The figure shows three views and two pictorial views of one solid part (mm, origin at its lowest corner). Answer the questions. Give positions to 0.01 mm unless a question says otherwise; leave off trailing zeros. Loops run counter-clockwise (first coordinate to the right, second up) from the corner with the lowest first, then second, coordinate; pieces in that order, holes last. Notation, with made-up numbers: (15.25, 34) -> (24.25, 34) arc R30 ccw to (24.25, 56) -> close; hole circle Ø5 at (57, 83.25). An arc over 180 degrees is marked (long way). Answer as CSV lines item,"result". Start each with the question number.
1. Find section A-A, the plane z = 1.55. Give the vertices of the cut face in (x, y).
2. A flat-ended cylindrical pin translates along its axis: pin 1 Ø1 at (x, z) = (2.5, 0.5) entering from +Y. Find the tip coordinate at first contact, or state that the pin passes through.
3. Find section B-B, the plane x = 10.75. Give the vertices of the cut face in (y, z).
4. Find the intervals of material crossed by line 1 along Y through (x, z) = (7, 2.25); line 2 along X through (y, z) = (41, 0.6); line 3 along Y through (x, z) = (2.75, 0.5), in increasing order.
5. Find section C-C, the plane x = 1. Give the vertices of the cut face in (y, z).
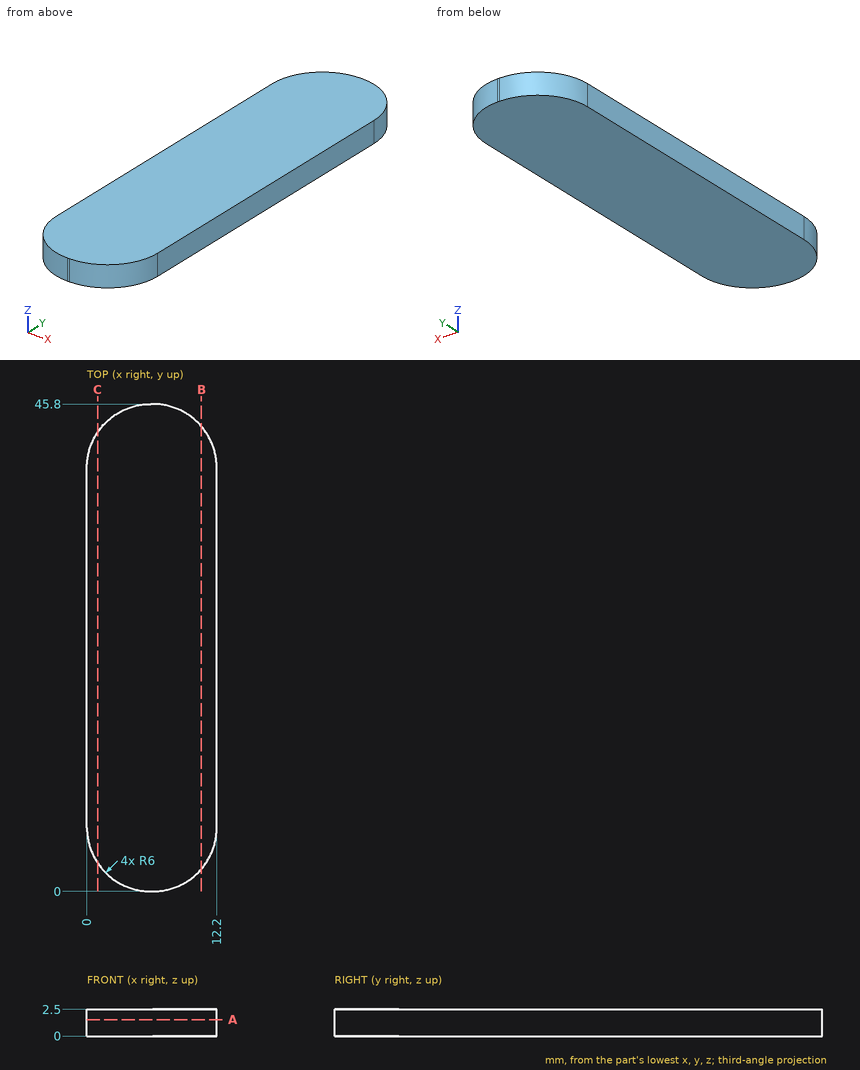
Resolved:
1,outline,"(0, 6) arc R6 ccw to (6, 0) -> (6.2, 0) arc R6 ccw to (12.2, 6) -> (12.2, 39.8) arc R6 ccw to (6.2, 45.8) -> (6, 45.8) arc R6 ccw to (0, 39.8) -> close"
2,pin 1,"stops at y = 45"
3,outline,"(2.09, 0) -> (43.71, 0) -> (43.71, 2.5) -> (2.09, 2.5) -> close"
4,line 1,"y = 0.05 to 45.75"
4,line 2,"x = 0.12 to 12.08"
4,line 3,"y = 0.96 to 44.84"
5,outline,"(2.68, 0) -> (43.12, 0) -> (43.12, 2.5) -> (2.68, 2.5) -> close"
